Source: three-view drawing plus pictorial views. Frame: mm from the lowest corner of the part. A direction names the side the tool comes from. Coordinates: 2 decimals unless noted, no trailing zeros. Write each loop counter-clockwise with the first axis right and the second up, starting at its lowest first coordinate (ties: lowest second). Pieces come first, ordered by that corner, then holes. Notation, with made-up numbers: M -32,0.5 L 7,0.5 A11 cw 7,10.5 Z; hole C -28,44 d2. An arc over 180 degrees is marked long. Write item = value, one per line. Start each with the question number.
Item 1: Section A-A on y = 4.7. Output: boundary loops of the cut face in (x, z) (1 decimal).
Item 2: First-contact query: pin 1 Ø2 at (y, z) = (2, 13) entering from +X (1 decimal); pin 2 Ø1.2 at (x, z) = (3, 5.5) entering from -Y (1 decimal); pin 3 Ø2.5 at (y, z) = (3, 7) entering from +X (1 decimal); pin 4 Ø2.5 at (x, y) = (3.5, 4) entering from -Z. Flat tips, straight axial feed; report the tip coordinate or a pass-through.
Item 3: Ray query, L1, parallel to Y at x = 2.9, z = 12.5 (1 decimal); L2, parallel to Z at x = 2.45, y = 2.5 (1 decimal); L3, parallel to Z at x = 0.6, y = 3. Return the intervals inside material, ascending. Write a range as [from, to].
Item 4: Section D-D on y = 3.85. Output: boundary loops of the cut face in (x, z) (1 decimal).
Item 5: Reachability of the marked faces 1, 2 and 3 from +Z, -Z, +X, -X, +Y, -Y: full face, straight path, thin tool, end or side. Return the list, or none.
Item 6: Pull-direction query (Z, two-part tool) for the marked faces 4 and 5; classes: +Z half, -Z half, draft (parallel to the pull), parting line (faces both ways), or undercut.
Item 7: Section B-B on x = 2.2. Give the number of separate pieces and of enclosed holes in the cut face.
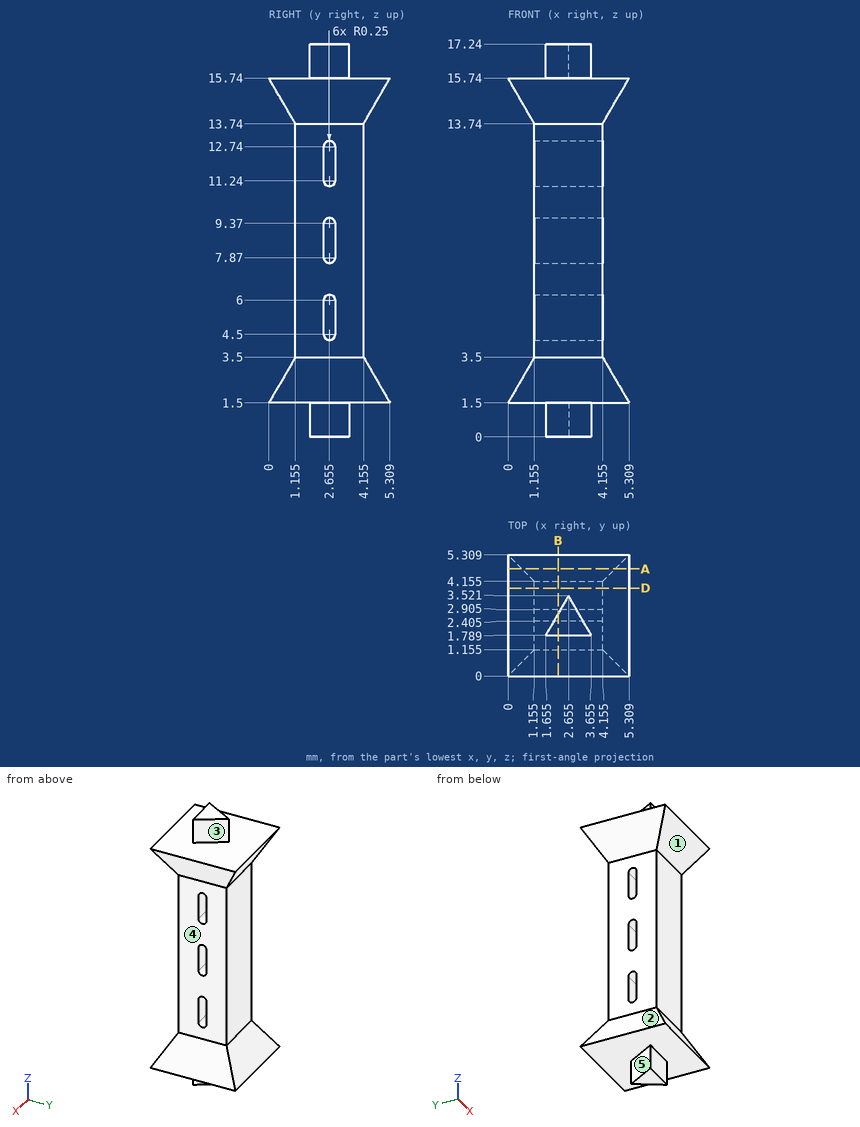
Responses:
q1.outline = M 0,1.5 L 5.3,1.5 L 4.7,2.6 L 0.6,2.6 Z; M 0,15.7 L 0.6,14.7 L 4.7,14.7 L 5.3,15.7 Z
q2.pin_1 = 4.3
q2.pin_2 = 1.2
q2.pin_3 = 4.2
q2.pin_4 = 0
q3.L1 = [1.2, 2.4], [2.9, 4.2]
q3.L2 = [0, 4.3], [6.2, 7.7], [9.6, 11], [12.9, 17.2]
q3.L3 = [1.5, 2.54], [14.7, 15.74]
q4.outline = M 0,1.5 L 5.3,1.5 L 4.2,3.5 L 4.2,13.7 L 5.3,15.7 L 0,15.7 L 1.2,13.7 L 1.2,3.5 Z
q5.face_1 = +X, -X, -Y
q5.face_2 = -X, +Y, -Y
q5.face_3 = +Z, +X, +Y
q6.face_4 = undercut
q6.face_5 = draft
q7.separate_pieces = 1
q7.enclosed_holes = 3
